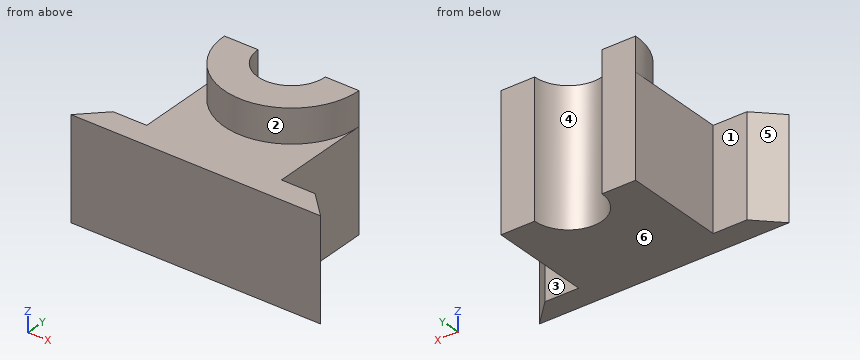
from build123d import *

# Parameters (mm, degrees)
BOSS_EXTRUDE1_DEPTH = 30
BOSS_EXTRUDE2_DEPTH = 40
CUT_EXTRUDE1_DEPTH  = 40


with BuildPart() as part:
    # Sketch1 → Boss-Extrude1 (new body)
    with BuildSketch(Plane.XY):
        Polygon((0, 0), (-10, 0), (-17.071067812, -7.071067812), (57.071067812, -7.071067812), (50, 0), (40, 0), (40, 30), (0, 30), align=None)
    extrude(amount=BOSS_EXTRUDE1_DEPTH)

    # Sketch3 → Boss-Extrude2 (add)
    with BuildSketch(Plane.XY):
        with BuildLine():
            Line((0, 30), (40, 30))
            ThreePointArc((40, 30), (20, 10), (0, 30))
        make_face()
    extrude(amount=BOSS_EXTRUDE2_DEPTH)

    # Sketch4 → Cut-Extrude1 (cut)
    with BuildSketch(Plane.XY.offset(40)):
        with BuildLine():
            Line((10, 30), (30, 30))
            ThreePointArc((30, 30), (20, 20), (10, 30))
        make_face()
    extrude(amount=-CUT_EXTRUDE1_DEPTH, mode=Mode.SUBTRACT)


solid = part.part
Read the model definition and answer for the solid it produces. Units are mm, in the model's axes. Face numbers are marked on the shaded views. A direction names the side the tool comes from. Give positions to 0.01 mm unless a question says otherwise; leave off trailing zeros. Write each loop counter-clockwise with the first axis right and the second up, starting at its lowest first coordinate (ties: lowest second). Pieces come first, ordered by that corner, then holes. Notation, with made-up numbers: (23, 21.25) - (29, 21.25) arc R33 cw to (29, 51.25) - close; hole circle Ø9 at (-6, -39.5). An arc over 180 degrees is marked (long way). Answer in a Markdown table with one row per item. Add a question column.
Item 1: Section C-C, the plane x = 20 is taken. Write down the section's boundary in (y, z).
Item 2: Section A-A, the plane y = 14 is taken. Write down the section's boundary in (x, z), and give its area (3 significant figures).
Item 3: A tool of negligible diameter and unlimited length cuts with its end or side. For the marked faces 1, 2 and 3, from which of +Z, -Z, +X, -X, +Y, -Y can it reach the whole face along a straight path? Write none if from no direction.
Item 4: Section D-D, the plane y = 26 is taken. Write down the section's boundary in (x, z), and give its area (3 significant figures).
Item 5: Section B-B, the plane z = 27.5 is taken. Write down the section's boundary in (x, y), and give its area (3 significant figures).
Item 6: Determine the mould class of the marked faces 4, 5 and 6 for opening direction X: pulls with the +X half, pulls with the -X half, needs draft (parallel to the pull), parting line crosses it, or undercut.
Item 7: Find the intervals of material crossed by L1, parallel to Y at x = 44, z = 14.5; L2, parallel to X at y = 15, z = 5; L3, parallel to Z at x = 34, y = 5, in increasing order.
Item 8: Flat-ended cylindrical pins translate along their axes: P1, Ø6, axis at x = 25.5, z = 17.5, coming from the +Y side; P2, Ø15, axis at y = 13, z = 10.5, coming from the +X side; P3, Ø5, axis at x = -2, y = 6.5, coming from the +Z side. Find the tip coordinate at first contact, or state that the pin passes through.
Recorded:
| question | item | result |
|---|---|---|
| 1 | outline | (-7.07, 0) - (20, 0) - (20, 40) - (10, 40) - (10, 30) - (-7.07, 30) - close |
| 2 | outline | (0, 0) - (40, 0) - (40, 30) - (32, 30) - (32, 40) - (8, 40) - (8, 30) - (0, 30) - close |
| 2 | area | 1,440 mm2 |
| 3 | face 1 | +Z, -Z, -X, +Y |
| 3 | face 2 | +Z, -Y |
| 3 | face 3 | +Z, -Z, +X, +Y |
| 4 | outline | (0, 0) - (10.83, 0) - (10.83, 40) - (0.4, 40) - (0.4, 30) - (0, 30) - close; (29.17, 0) - (40, 0) - (40, 30) - (39.6, 30) - (39.6, 40) - (29.17, 40) - close |
| 4 | area | 859 mm2 |
| 5 | outline | (-17.07, -7.07) - (57.07, -7.07) - (50, 0) - (40, 0) - (40, 30) - (30, 30) arc R10 cw to (10, 30) - (0, 30) - (0, 0) - (-10, 0) - close |
| 5 | area | 1,520 mm2 |
| 6 | face 4 | undercut |
| 6 | face 5 | pulls with the -X half |
| 6 | face 6 | needs draft |
| 7 | L1 | y = -7.07 to 0 |
| 7 | L2 | x = 0 to 40 |
| 7 | L3 | z = 0 to 30 |
| 8 | P1 | stops at y = 24.73 |
| 8 | P2 | stops at x = 40 |
| 8 | P3 | stops at z = 30 |
